Geometry check sheet. Reference: the model listing, model coordinates, mm. Face numbers are marked on the shaded views. Round coordinates to 2 decimals unless told otherwise and drop trailing zeros. Loops run counter-clockwise (first coordinate to the right, second up) from the corner with the lowest first, then second, coordinate; pieces in that order, holes last. Notation, with made-up numbers: (-30.5, 89.5) - (-4.5, 89.5) arc R30 cw to (-4.5, 119.5) - close; hole circle Ø9 at (-20.75, 60.5). An arc over 180 degrees is marked (long way). Answer as CSV lines item,"result". Start each with the question number.
1) Cross-section at C-C on z = -76.5. Record the boundary of the cut face in (x, y).
2) Draft check along X on the marked faces 1, 2, 3 and 4. Enter one of: released by +X, released by -X, zero draft, split by the parting line, or undercut.
3) Thickness scan on line 1 along Z through (x, y) = (4, 71); line 2 along X through (y, z) = (28, 38.5); line 3 along Y through (x, z) = (84, 39). Record the ranges inside material, lowest first.
4) Cross-section at D-D on x = -116. Record the boundary of the cut face in (y, z).
5) Cross-section at B-B on y = 45. Record the boundary of the cut face in (x, z).
6) Depth check by flat-ended pin: P1, Ø6, axis at y = 88, z = 95.5, coming from the +X side; P2, Ø1.5, axis at y = 84.5, z = 39, coming from the +X side; P3, Ø4, axis at x = -129, y = 20.5, coming from the +Z side. Enter the tip coordinate at first touch or a pass-through.
7) Cross-section at A-A on x = 134. Record the boundary of the cut face in (y, z).
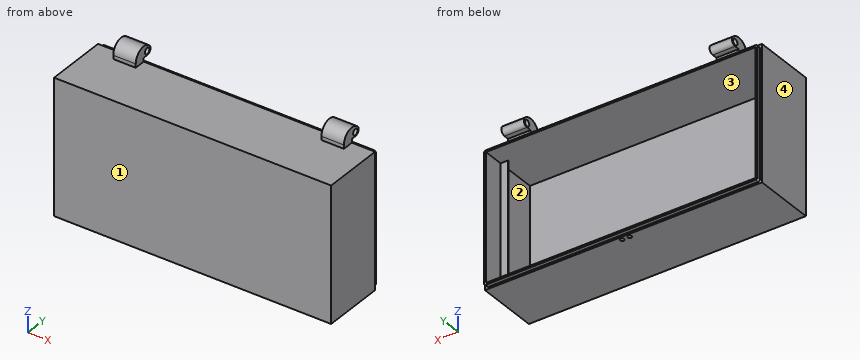
from build123d import *

# Parameters (mm, degrees)
BOSS_EXTRUDE1_DEPTH     = 85
SKETCH3_W               = 370
SKETCH3_H               = 5
BOSS_EXTRUDE2_DEPTH     = 87.5
SKETCH4_W               = 2.5
SKETCH4_H               = 5
CUT_EXTRUDE1_DEPTH      = 391.712490202
CUT_EXTRUDE2_DEPTH      = 271.90127353
CUT_EXTRUDE2_DEPTH_BACK = 271.90127353
SKETCH5_W               = 2.5
SKETCH5_H               = 5
FILLET1_R               = 2.5
SKETCH6_W               = 10
SKETCH6_H               = 170
BOSS_EXTRUDE3_DEPTH     = 10
FILLET2_SIZE            = 9
SKETCH8_W               = 30
SKETCH8_H               = 15
REVOLVE1_ANGLE          = 180
FILLET9_R               = 6
SKETCH12_W              = 5
SKETCH12_H              = 15
BOSS_EXTRUDE5_DEPTH     = 30
SKETCH9_R               = 4.1
CUT_EXTRUDE4_DEPTH      = 370.495940438
FILLET11_R              = 6
SKETCH13_R              = 2.5
CUT_EXTRUDE5_DEPTH      = 30


with BuildPart() as part:
    # Sketch2 → Boss-Extrude1 (new, symmetric)
    with BuildSketch(Plane.XY):
        Polygon((-185, 0), (185, 0), (185, 82.5), (182.5, 82.5), (182.5, 87.5), (180, 87.5), (180, 80.5), (180, 5), (-180, 5), (-180, 80.5), (-180, 87.5), (-182.5, 87.5), (-182.5, 82.5), (-185, 82.5), align=None)
    extrude(amount=BOSS_EXTRUDE1_DEPTH, both=True)

    # Sketch3 → Boss-Extrude2 (add)
    with BuildSketch(Plane(origin=(0, 0, 0), x_dir=(1, 0, 0), z_dir=(0, 1, 0))):
        with Locations((0, -87.5)):
            Rectangle(SKETCH3_W, SKETCH3_H)
        with Locations((0, 87.5)):
            Rectangle(SKETCH3_W, SKETCH3_H)
    extrude(amount=BOSS_EXTRUDE2_DEPTH)

    # Sketch4 → Cut-Extrude1 (cut, through all)
    with BuildSketch(Plane(origin=(185, 0, 0), x_dir=(0, 0, -1), z_dir=(1, 0, 0))):
        with Locations((-88.75, 85)):
            Rectangle(SKETCH4_W, SKETCH4_H)
        with Locations((88.75, 85)):
            Rectangle(SKETCH4_W, SKETCH4_H)
    extrude(amount=-CUT_EXTRUDE1_DEPTH, mode=Mode.SUBTRACT)

    # Sketch5 → Cut-Extrude2 (cut, two sides: drawn at the far end of the back side and taken through both)
    with BuildSketch(Plane(origin=(0, 0, -87.5), x_dir=(-1, 0, 0), z_dir=(0, 0, -1)).offset(-CUT_EXTRUDE2_DEPTH_BACK)):
        with Locations((-183.75, 85)):
            Rectangle(SKETCH5_W, SKETCH5_H)
        with Locations((183.75, 85)):
            Rectangle(SKETCH5_W, SKETCH5_H)
    extrude(amount=CUT_EXTRUDE2_DEPTH + CUT_EXTRUDE2_DEPTH_BACK, mode=Mode.SUBTRACT)

    # Fillet1
    fillet1_edges = [part.edges().sort_by_distance(p)[0] for p in [
        (182.5, 85, 87.5),
        (182.5, 85, -87.5),
        (-182.5, 85, 87.5),
        (-182.5, 85, -87.5),
    ]]
    fillet(fillet1_edges, radius=FILLET1_R)

    # Sketch6 → Boss-Extrude3 (add)
    with BuildSketch(Plane(origin=(0, 60, 0), x_dir=(1, 0, 0), z_dir=(0, 1, 0))):
        with Locations((-175, 0)):
            Rectangle(SKETCH6_W, SKETCH6_H)
        with Locations((175, 0)):
            Rectangle(SKETCH6_W, SKETCH6_H)
    extrude(amount=-BOSS_EXTRUDE3_DEPTH)

    # Fillet2
    fillet2_edges = [part.edges().sort_by_distance(p)[0] for p in [
        (-170, 50, 0),
        (170, 50, 0),
    ]]
    chamfer(fillet2_edges, length=FILLET2_SIZE)



with BuildPart() as body_2:
    # Sketch8 → Revolve1 (revolve, symmetric)
    with BuildSketch(Plane(origin=(0, 82.5, 0), x_dir=(1, 0, 0), z_dir=(0, 1, 0))) as revolve1_sk:
        with Locations((-139, -102.5)):
            Rectangle(SKETCH8_W, SKETCH8_H)
    revolve1 = revolve(axis=Axis((184.702128339, 82.5, 95), (-1, 0, 0)), revolution_arc=REVOLVE1_ANGLE / 2)
    revolve1 = revolve1 + revolve(revolve1_sk.sketch, axis=Axis((184.702128339, 82.5, 95), (1, 0, 0)), revolution_arc=REVOLVE1_ANGLE / 2)

    # Fillet9
    fillet9_edges = [body_2.edges().sort_by_distance(p)[0] for p in [
        (-139, 97.5, 95),
    ]]
    fillet(fillet9_edges, radius=FILLET9_R)


with BuildPart() as part_1:
    add(part.part)

    add(body_2.part)  # Boss-Extrude5 merges body 2
    # Sketch12 → Boss-Extrude5 (add)
    with BuildSketch(Plane.ZY.offset(154)):
        with Locations((92.5, 75)):
            Rectangle(SKETCH12_W, SKETCH12_H)
    boss_extrude5 = extrude(amount=-BOSS_EXTRUDE5_DEPTH)

    # Mirror4: Boss-Extrude5 across plane
    add(boss_extrude5.mirror(Plane(origin=(0, 0, 0), x_dir=(0, 0, 1), z_dir=(1, 0, 0))))

    # Mirror5: Revolve1 across plane
    add(revolve1.mirror(Plane(origin=(0, 0, 0), x_dir=(0, 0, 1), z_dir=(1, 0, 0))))

    # Sketch9 → Cut-Extrude4 (cut, through all)
    with BuildSketch(Plane.ZY.offset(154)):
        with Locations(Location((100.5, 89, 0), (0, 0, 180))):
            Circle(SKETCH9_R)
    extrude(amount=-CUT_EXTRUDE4_DEPTH, mode=Mode.SUBTRACT)

    # Fillet11
    fillet11_edges = [part_1.edges().sort_by_distance(p)[0] for p in [
        (139, 97.5, 95),
    ]]
    fillet(fillet11_edges, radius=FILLET11_R)

    # Sketch13 → Cut-Extrude5 (cut)
    with BuildSketch(Plane(origin=(0, 0, -90), x_dir=(-1, 0, 0), z_dir=(0, 0, -1))):
        with Locations((-5, 77.5)):
            Circle(SKETCH13_R)
        with Locations((5, 77.5)):
            Circle(SKETCH13_R)
    extrude(amount=-CUT_EXTRUDE5_DEPTH, mode=Mode.SUBTRACT)


solid = part_1.part
Answer block:
1,outline,"(-185, 0) - (185, 0) - (185, 82.5) - (182.5, 82.5) - (182.5, 87.5) - (180, 87.5) - (180, 60) - (170, 60) - (170, 59) - (179, 50) - (180, 50) - (180, 5) - (-180, 5) - (-180, 50) - (-179, 50) - (-170, 59) - (-170, 60) - (-180, 60) - (-180, 87.5) - (-182.5, 87.5) - (-182.5, 82.5) - (-185, 82.5) - close"
2,face 1,"zero draft"
2,face 2,"undercut"
2,face 3,"undercut"
2,face 4,"released by -X"
3,line 1,"z = -90 to -85, 85 to 90"
3,line 2,"x = -185 to -180, 180 to 185"
3,line 3,"y = 0 to 5"
4,outline,"(0, -90) - (82.5, -90) - (82.5, -87.5) - (87.5, -87.5) - (87.5, -85) - (5, -85) - (5, 85) - (87.5, 85) - (87.5, 87.5) - (82.5, 87.5) - (82.5, 90) - (0, 90) - close"
5,outline,"(-185, -90) - (185, -90) - (185, 90) - (-185, 90) - close; hole (-180, -85) - (180, -85) - (180, 85) - (-180, 85) - close"
6,P1,"stops at x = 154"
6,P2,"stops at x = 182.5"
6,P3,"stops at z = 90"
7,outline,"(0, -90) - (82.5, -90) - (82.5, -87.5) - (87.5, -87.5) - (87.5, -85) - (5, -85) - (5, 85) - (87.5, 85) - (87.5, 87.5) - (82.5, 87.5) - (82.5, 95) - (89.21, 95) arc R6 ccw to (93.68, 105) arc R15 ccw to (67.5, 95) - (67.5, 90) - (0, 90) - close; hole circle Ø8.2 at (89, 100.5)"
